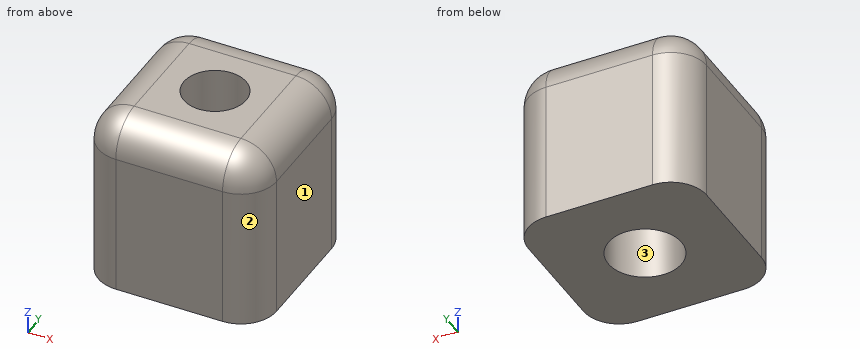
from build123d import *

# Parameters (mm, degrees)
SKETCH1_W           = 10
SKETCH1_H           = 10
BOSS_EXTRUDE1_DEPTH = 10
SKETCH2_R           = 1.75
CUT_EXTRUDE1_DEPTH  = 11
SKETCH3_R           = 2.05
CUT_EXTRUDE2_DEPTH  = 5
FILLET1_R           = 2
FILLET2_R           = 2


with BuildPart() as part:
    # Sketch1 → Boss-Extrude1 (new body)
    with BuildSketch(Plane.XY):
        with Locations((5, 5)):
            Rectangle(SKETCH1_W, SKETCH1_H)
    extrude(amount=BOSS_EXTRUDE1_DEPTH)

    # Sketch2 → Cut-Extrude1 (cut, through all)
    with BuildSketch(Plane.XY.offset(10)):
        with Locations((5, 5)):
            Circle(SKETCH2_R)
    extrude(amount=-CUT_EXTRUDE1_DEPTH, mode=Mode.SUBTRACT)

    # Sketch3 → Cut-Extrude2 (cut)
    with BuildSketch(Plane(origin=(0, 0, 0), x_dir=(-1, 0, 0), z_dir=(0, 0, -1))):
        with Locations((-5, 5)):
            Circle(SKETCH3_R)
    extrude(amount=-CUT_EXTRUDE2_DEPTH, mode=Mode.SUBTRACT)

    # Fillet1
    fillet1_edges = [part.edges().sort_by_distance(p)[0] for p in [
        (0, 10, 5),
        (10, 10, 5),
        (10, 0, 5),
        (0, 0, 5),
    ]]
    fillet(fillet1_edges, radius=FILLET1_R)

    # Fillet2
    fillet2_edges = [part.edges().sort_by_distance(p)[0] for p in [
        (5, 10, 10),
        (10, 5, 10),
        (0, 5, 10),
        (5, 0, 10),
        (9.414213562, 0.585786438, 10),
        (0.585786438, 0.585786438, 10),
        (0.585786438, 9.414213562, 10),
        (9.414213562, 9.414213562, 10),
    ]]
    fillet(fillet2_edges, radius=FILLET2_R)


solid = part.part
Work out the finished part from the listing and answer in its coordinate system (mm). Face numbers are marked on the shaded views. Coordinates: 2 decimals unless noted, no trailing zeros. Write each loop counter-clockwise with the first axis right and the second up, starting at its lowest first coordinate (ties: lowest second). Pieces come first, ordered by that corner, then holes. Notation, with made-up numbers: M 25.25,-35 L 44.25,-35 A20 cw 44.25,-13 Z; hole C 7,76.5 d3. An arc over 180 degrees is marked long. Use one line per item in the form item = value. Start each with the question number.
1. The part is cut by section D-D (x = 2.75). Give the vertices of the cut face in (y, z), plus the area to 3 significant figures.
2. Straight lines are drawn through the part: probe 1 along Y at (x, z) = (5, 7.8); probe 2 along Y at (x, z) = (5, 2.7); probe 3 along X at (y, z) = (4.25, 0.5). For each, find the intervals that lie inside material, in ascending order. Write a range as from..to.
3. The part is cut by section C-C (z = 3.5). Give the vertices of the cut face in (x, y).
4. The mould has two halves that part along Y. Classify the marked faces 1, 2 and 3: released by +Y, released by -Y, zero draft, split by the parting line, or undercut.
5. The part is cut by section A-A (y = 5). Give the vertices of the cut face in (x, z), plus the area to 3 significant figures.
Evaluation:
q1.outline = M 0,0 L 10,0 L 10,8 A2 ccw 8,10 L 2,10 A2 ccw 0,8 Z
q1.area = 98.3 mm^2
q2.probe_1 = 0..3.25, 6.75..10
q2.probe_2 = 0..2.95, 7.05..10
q2.probe_3 = 0..3.09, 6.91..10
q3.outline = M 0,2 A2 ccw 2,0 L 8,0 A2 ccw 10,2 L 10,8 A2 ccw 8,10 L 2,10 A2 ccw 0,8 Z; hole C 5,5 d4.1
q4.face_1 = zero draft
q4.face_2 = released by -Y
q4.face_3 = undercut
q5.outline = M 0,0 L 2.95,0 L 2.95,5 L 3.25,5 L 3.25,10 L 2,10 A2 ccw 0,8 Z; M 6.75,5 L 7.05,5 L 7.05,0 L 10,0 L 10,8 A2 ccw 8,10 L 6.75,10 Z
q5.area = 60.3 mm^2
